```python
from build123d import *

# Parameters (mm, degrees)
SKETCH001_R   = 5.5
POCKET_DEPTH  = 2.001
FILLET_R      = 2
CHAMFER_SIZE2 = 1.5
CHAMFER_SIZE  = 1


with BuildPart() as part:
    # Sketch → Revolution (revolve)
    with BuildSketch(Plane.XZ):
        Polygon((0, 0), (0, 2), (14.25, 2), (14.25, 20), (16.25, 20), (19, 0), align=None)
    revolve(axis=Axis((0, 0, 0), (0, 0, 1)))

    # Sketch001 (on Face1 of Revolution) → Pocket (cut, through all)
    with BuildSketch(Plane(origin=(0, 0, 2), x_dir=(-1, 0, 0), z_dir=(0, 0, 1))):
        with Locations((0, -2)):
            Circle(SKETCH001_R)
        with BuildLine():
            ThreePointArc((2, 8), (0, 10), (-2, 8))
            Line((-2, 8), (-2, -2))
            ThreePointArc((-2, -2), (0, -4), (2, -2))
            Line((2, 8), (2, -2))
        make_face()
    extrude(amount=-POCKET_DEPTH, mode=Mode.SUBTRACT)

    # Fillet
    fillet_edges = [part.edges().sort_by_distance(p)[0] for p in [
        (-16.25, 0, 20),
    ]]
    fillet(fillet_edges, radius=FILLET_R)

    # Chamfer
    chamfer_edges = [part.edges().sort_by_distance(p)[0] for p in [
        (-4.541476, -1.102418, 2),
        (3.102418, 6.541476, 2),
        (2, -5.561738, 2),
        (0, -10, 2),
        (-2, -5.561738, 2),
    ]]
    chamfer_side = part.faces().sort_by_distance((-13.846949, 0, 2))[0]
    chamfer(chamfer_edges, length=CHAMFER_SIZE, length2=CHAMFER_SIZE2, reference=chamfer_side)


solid = part.part
```
Could you check a few things on this model? Use its own coordinates, in mm. A direction names the side the tool comes from. Give positions to 0.01 mm unless a question says otherwise; leave off trailing zeros. Loops run counter-clockwise (first coordinate to the right, second up) from the corner with the lowest first, then second, coordinate; pieces in that order, holes last. Notation, with made-up numbers: (74.5, 52.5) - (96.5, 52.5) arc R18 cw to (96.5, 64.5) - close; hole circle Ø5 at (46.25, 65). An arc over 180 degrees is marked (long way). Answer in a Markdown table with one row per item. Add a question column.
Q1. If we section it at A-A (x = 0): List the corners of the cut face in (y, z) for me, plus the area to 3 significant figures.
Q2. Which directions (+Z, -Z, +X, -X, +Y, -Y) give clear straight access to the entire face, cutting with the end or side of a thin tool? Please do faces 4 (the face through (7, 0, 2)), 5 (the face through (0, -10, 0.3)).
Q3. If we section it at B-B (z = 12): List the corners of the cut face in (x, y) for me.
Q4. If we section it at C-C (z = 1.5): List the corners of the cut face in (x, y) for me.
Q5. For pin 1 (12 mm diameter, centred on y = 10.5, z = 13.5, fed in from +X); pin 2 (3 mm diameter, centred on y = 9.5, z = 16, fed in from +X); pin 3 (14 mm diameter, centred on x = 3.5, y = 0, fed in from +Z), each with a flat end and sliding along its axis, tell me the tip position at first contact or that it passes through.
Q6. Please list where these lines run through material, in increasing order: L1, parallel to Y at x = 0, z = 15.5; L2, parallel to Y at x = 0, z = 0.2; L3, parallel to X at y = -5.5, z = 6.75. Write a range as from..to.
Q7. We'd pull the mould along Y, two halves only. Please class faces 1 (the face through (-13.87, -10.64, 11.04)), 2 (the face through (0.213, 7.496, 0.254)), 3 (the face through (4, -4, 0)): +Y half, -Y half, draft (parallel to the pull), parting line (faces both ways), or undercut.
The answers:
| question | item | result |
|---|---|---|
| 1 | outline | (-19, 0) - (-10, 0) - (-10, 0.5) - (-11, 2) - (-14.25, 2) - (-14.25, 20) - (-14.51, 20) arc R2 ccw to (-16.49, 18.27) - close; (7.5, 0) - (19, 0) - (16.49, 18.27) arc R2 ccw to (14.51, 20) - (14.25, 20) - (14.25, 2) - (8.5, 2) - (7.5, 0.5) - close |
| 1 | area | 154 mm^2 |
| 2 | face 4 | +Z |
| 2 | face 5 | +Z, -Z |
| 3 | outline | circle Ø34.7 at (0, 0); hole circle Ø28.5 at (0, 0) |
| 4 | outline | circle Ø37.59 at (0, 0); hole (-2.67, -8) arc R2.67 ccw to (2.67, -8) - (2.67, -3.56) arc R6.17 ccw (long way) to (-2.67, -3.56) - close |
| 5 | pin 1 | stops at x = 16.74 |
| 5 | pin 2 | stops at x = 14.81 |
| 5 | pin 3 | stops at z = 2 |
| 6 | L1 | y = -16.87..-14.25, 14.25..16.87 |
| 6 | L2 | y = -18.97..-10, 7.5..18.97 |
| 6 | L3 | x = -17.21..-13.15, 13.15..17.21 |
| 7 | face 1 | parting line |
| 7 | face 2 | undercut |
| 7 | face 3 | draft |
